Autodesk Fusion 360 part; units mm, degrees
sketch "Sketch1" plane through (0, 0, 0) normal (0, 0, 1) x (1, 0, 0)
  line L0 (17.5, -25) -> (-17.5, -25)
  line L1 (5.5, -23) -> (-5.5, -23)
  line L2 (-5.5, -23) -> (-5.5, -16)
  line L3 (-5.5, -16) -> (5.5, -16)
  line L4 (5.5, -16) -> (5.5, -23)
  line L5 (-24.2785, 8.8924) -> (-22.4011, 8.8924)
  line L6 (-17.5, -25) -> (-24.2785, 8.8924)
  line L7 (22.4011, 8.8924) -> (24.2781, 8.8924)
  line L8 (24.2781, 8.8924) -> (17.5, -25)
  arc A0 (-22.4011, 8.8924) -> (22.4011, 8.8924) centre (0, 11) ccw
  dimension "d4" = 45
  dimension "d5" = 1.877
extrude "Extrude1" add sketch "Sketch1" along normal blind 120
extrude "Extrude2" add sketch "Sketch1" along normal blind 120 contours L1 L2 L3 L4
extrude "Extrude3" cut sketch "Sketch1" along normal blind 20 contours L1 L2 L3 L4
sketch "Sketch2" plane through (0, 0, 120) normal (0, 0, 1) x (-1, 0, 0)
  line L0 (22.4011, -8.8924) -> (24.2785, -8.8924)
  line L1 (24.2785, -8.8924) -> (17.5, 25)
  line L2 (17.5, 25) -> (-17.5, 25)
  line L3 (-17.5, 25) -> (-24.2781, -8.8924)
  line L4 (-24.2781, -8.8924) -> (-22.4011, -8.8924)
  arc A0 (22.4011, -8.8924) -> (-22.4011, -8.8924) centre (0, -11) ccw
  line L5 (-5.5, 23) -> (5.5, 23)
  line L6 (5.5, 23) -> (5.5, 16)
  line L7 (5.5, 16) -> (-5.5, 16)
  line L8 (-5.5, 16) -> (-5.5, 23)
extrude "Extrude4" add sketch "Sketch2" along normal blind 20 contours L5 L6 L7 L8
sketch "Sketch3" plane through (0, 0, 0) normal (0, 0, 1) x (1, 0, 0)
  circle A0 centre (0, 10) radius 27.8887
  line L0 (-10.2931, -15.9198) -> (-10.2931, -26.4867)
  line L1 (-10.2931, -26.4867) -> (10, -26.4867)
  line L2 (10, -26.4867) -> (10, -16.0342)
  line L3 (-10.2931, -26.4867) -> (-25, -26.4867)
  line L4 (-25, -26.4867) -> (-25, -2.3605)
  line L5 (10, -26.4867) -> (25, -26.4867)
  line L6 (25, -26.4867) -> (25, -2.3605)
extrude "Extrude5" cut sketch "Sketch3" along normal blind 135 contours A0 L0 L3 L4 | A0 L2 L5 L6
Geometry: final body of the model. Coordinates: model frame, mm. A direction names the side the tool comes from. Coordinates: 2 decimals unless noted, no trailing zeros. Order: outer loops, then holes, each group sorted by start corner. A loop starts at its lowest first (then second) coordinate and runs counter-clockwise, first axis right, second up. Notation, with made-up numbers: M -3,87.25 L 21,87.25 A22 ccw 21,96.25 Z; hole C 74,84.5 d7. An arc over 180 degrees is marked long. Answer in a Markdown table with one row per item. Add a question column.
Q1. Section query C-C on z = 68.5. Return the cut outline in (x, y), and give its area (3 significant figures).
Q2. Section query B-B on z = 12. Return the cut outline in (x, y).
Q3. Contact query for flat-ended pins moving along their axis: P1, Ø3.5, axis at x = -1, y = -18.5, coming from the -Z side; P2, Ø2, axis at y = -20.5, z = 24.5, coming from the -X side; P3, Ø2, axis at x = 16.5, z = 102, coming from the -Y side. Output: stop coordinate, or through.
Q4. Section query D-D on x = 2.5. Return the cut outline in (y, z), and give its area (3 significant figures).
Q5. Line query: L1, parallel to X at y = -18.5, z = 18.5; L2, parallel to X at y = -17, z = 65; L3, parallel to X at y = 5, z = 116.5. Output: solid intervals per line, ascending.
Q6. Mould query, pull axis Y, two halves, no side actions, for faces 5 (the cylindrical face through (0.465, -11.495, 59.16)), 6 (the flat face through (5.5, -19, 10)), 7 (the flat face through (-5.5, -20, 10)), 8 (the flat face through (-5.5, -20, 130)). Classes: released by +Y, released by -Y, zero draft, split by the parting line, or undercut.
Q7. Section query A-A on y = 3.5. Return the cut outline in (x, z).
Q8. Reachability of faces 1 (the flat face through (-10.293, -20, 59)), 2 (the flat face through (10, -21, 59)), 3 (the flat face through (0, -23, 10)), 4 (the flat face through (0, -16, 130)) from +Z, -Z, +X, -X, +Y, -Y: full face, straight path, thin tool, end or side. Return the list, or none.
Completed:
| question | item | result |
|---|---|---|
| 1 | outline | M -24.28,8.89 L -20.78,-8.6 A27.89 ccw -10.29,-15.92 L -10.29,-25 L 10,-25 L 10,-16.03 A27.89 ccw 20.78,-8.6 L 24.28,8.89 L 22.4,8.89 A22.5 cw -22.4,8.89 Z |
| 1 | area | 512 mm2 |
| 2 | outline | M -24.28,8.89 L -20.78,-8.6 A27.89 ccw -10.29,-15.92 L -10.29,-25 L 10,-25 L 10,-16.03 A27.89 ccw 20.78,-8.6 L 24.28,8.89 L 22.4,8.89 A22.5 cw -22.4,8.89 Z; hole M -5.5,-23 L 5.5,-23 L 5.5,-16 L -5.5,-16 Z |
| 3 | P1 | stops at z = 20 |
| 3 | P2 | stops at x = -10.29 |
| 3 | P3 | stops at y = -13.18 |
| 4 | outline | M -25,0 L -23,0 L -23,20 L -16,20 L -16,0 L -11.36,0 L -11.36,120 L -16,120 L -16,140 L -23,140 L -23,120 L -25,120 Z |
| 4 | area | 1,640 mm2 |
| 5 | L1 | x = -10.29 to -5.5, 5.5 to 10 |
| 5 | L2 | x = -10.29 to 10 |
| 5 | L3 | x = -23.5 to -21.69, 21.69 to 23.5 |
| 6 | face 5 | released by +Y |
| 6 | face 6 | undercut |
| 6 | face 7 | undercut |
| 6 | face 8 | zero draft |
| 7 | outline | M -23.2,0 L -21.21,0 L -21.21,120 L -23.2,120 Z; M 21.21,0 L 23.2,0 L 23.2,120 L 21.21,120 Z |
| 8 | face 1 | +Z, -Z, -X, -Y |
| 8 | face 2 | +Z, -Z, +X, -Y |
| 8 | face 3 | -Z |
| 8 | face 4 | +Z, +X, -X, +Y |
